from build123d import *

# Parameters (mm, degrees)
SKETCH1_W            = 76.5658
SKETCH1_H            = 16.378
BASE_FLANGE1_DEPTH   = 3.175
M6_CLEARANCE_HOLE1_D = 6.6
FILLET1_R            = 2.54


# Sheet-metal steps are written as plain solids
with BuildPart() as part:
    # Sketch1 → Base-Flange1 (new body)
    with BuildSketch(Plane.XY):
        with Locations((15.489, -70.312600001)):
            Rectangle(SKETCH1_W, SKETCH1_H)
    extrude(amount=-BASE_FLANGE1_DEPTH)

    # M6 Clearance Hole1 (through all)
    with Locations(Plane.XY):
        with Locations((-14.4119, -70.312600001), (45.5829, -70.312600001)):
            Hole(M6_CLEARANCE_HOLE1_D / 2)

    # Fillet1
    fillet1_edges = [part.edges().sort_by_distance(p)[0] for p in [
        (-22.7939, -62.123600001, -1.5875),
        (53.7719, -62.123600001, -1.5875),
        (53.7719, -78.501600001, -1.5875),
        (-22.7939, -78.501600001, -1.5875),
    ]]
    fillet(fillet1_edges, radius=FILLET1_R)


solid = part.part
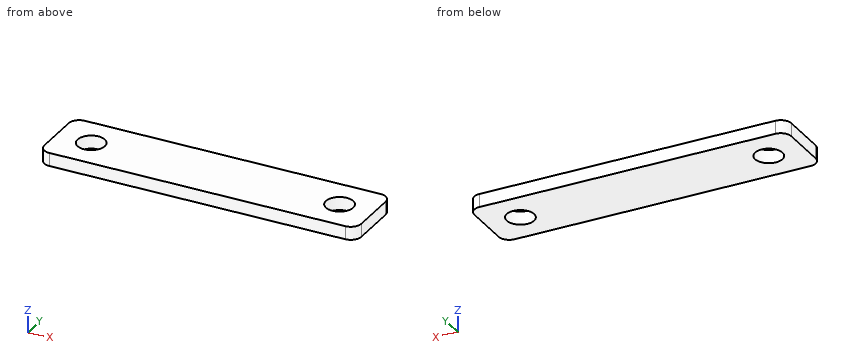
Could you check a few things on this model? Use its own coordinates, in mm. Give positions to 0.01 mm unless a question says otherwise; leave off trailing zeros. Write each loop counter-clockwise with the first axis right and the second up, starting at its lowest first coordinate (ties: lowest second). Pieces come first, ordered by that corner, then holes. Notation, with made-up numbers: (-3, 26) -> (12, 26) arc R12 cw to (12, 48) -> close; hole circle Ø4 at (-37, 30). An arc over 180 degrees is marked (long way). Answer as a JSON object with one key per item and string values.
Q1. Will this pin go through, and if not, where does the flat tip stop? pin 1 Ø4 at (x, y) = (45.58, -70.31) entering from +Z.
Taken from the geometry:
{"pin 1": "passes through"}
Q2. Suppose I cut it at C-C on z = -0.7. Write out the boundary of the cut face in (x, y).
Taken from the geometry:
{"outline": "(-22.79, -75.96) arc R2.54 ccw to (-20.25, -78.5) -> (51.23, -78.5) arc R2.54 ccw to (53.77, -75.96) -> (53.77, -64.66) arc R2.54 ccw to (51.23, -62.12) -> (-20.25, -62.12) arc R2.54 ccw to (-22.79, -64.66) -> close; hole circle Ø6.6 at (-14.41, -70.31); hole circle Ø6.6 at (45.58, -70.31)"}
Q3. Suppose I cut it at B-B on x = 45.5. Write out the boundary of the cut face in (y, z) (3 decimals), then the cut area to 3 significant figures.
Taken from the geometry:
{"outline": "(-78.502, -3.175) -> (-73.612, -3.175) -> (-73.612, 0) -> (-78.502, 0) -> close; (-67.014, -3.175) -> (-62.124, -3.175) -> (-62.124, 0) -> (-67.014, 0) -> close", "area": "31.1 mm²"}
Q4. Suppose I cut it at A-A on y = -71. Write out the boundary of the cut face in (x, z) (3 decimals).
Taken from the geometry:
{"outline": "(-22.794, -3.175) -> (-17.64, -3.175) -> (-17.64, 0) -> (-22.794, 0) -> close; (-11.184, -3.175) -> (42.355, -3.175) -> (42.355, 0) -> (-11.184, 0) -> close; (48.811, -3.175) -> (53.772, -3.175) -> (53.772, 0) -> (48.811, 0) -> close"}
Q5. Please list where these lines run through material, in increasing order: L1, parallel to X at y = -72.25, z = -0.8; L2, parallel to X at y = -71, z = -0.6; L3, parallel to X at y = -64.5, z = -1.75.
Taken from the geometry:
{"L1": "x = -22.79 to -17.08, -11.74 to 42.91, 48.25 to 53.77", "L2": "x = -22.79 to -17.64, -11.18 to 42.36, 48.81 to 53.77", "L3": "x = -22.79 to 53.77"}
Q6. Suppose I cut it at D-D on x = -12. Write out the boundary of the cut face in (y, z) (3 decimals), then the cut area to 3 significant figures.
Taken from the geometry:
{"outline": "(-78.502, -3.175) -> (-72.565, -3.175) -> (-72.565, 0) -> (-78.502, 0) -> close; (-68.06, -3.175) -> (-62.124, -3.175) -> (-62.124, 0) -> (-68.06, 0) -> close", "area": "37.7 mm²"}
